Build history of the part. All positions in model axes, mm. Face numbers are marked on the shaded views. A direction names the side the tool comes from. Round coordinates to 2 decimals unless told otherwise and drop trailing zeros. Write each loop counter-clockwise with the first axis right and the second up, starting at its lowest first coordinate (ties: lowest second). Pieces come first, ordered by that corner, then holes.
Item 1: Band-saw the part on C-C, the plane x = -3. Write the cut outline in (y, z).
Item 2: Band-saw the part on A-A, the plane y = -2. Write the cut outline in (x, z).
Item 3: Wall check: probe 1 along Y at (x, z) = (0, 53.75); probe 2 along X at (y, z) = (0, 55.5); probe 3 along Z at (x, y) = (5.5, 1.25). Give the ranges that are in metal, low to high.
Item 4: 3-axis set-ups, long thin cutter, end or side, ignore diameter. For the marked faces 1 and 2: which of +Z, -Z, +X, -X, +Y, -Y reach the whole face in a straight line?
Item 5: Drop flat-ended pins along their axis: pin 1 Ø1 at (y, z) = (0.5, 33) entering from +X; pin 2 Ø1.5 at (y, z) = (5, 49) entering from -X; pin 3 Ø2 at (y, z) = (-2, 10.5) entering from -X. Give the stop position or say it passes through.
Item 6: Band-saw the part on B-B, the plane z = 13. Write the cut outline in (x, y), then the cut area to 3 significant figures.
Autodesk Inventor part; units mm, degrees
ref_plane "作業平面1" through (0, 6, 58.85) normal (0, 1, 0) x (-1, 0, 0)
ref_plane "YZ Plane" through (0, 0, 0) normal (1, 0, 0) x (0, 1, 0)
ref_plane "XZ Plane" through (0, 0, 0) normal (0, 1, 0) x (-1, 0, 0)
sketch "スケッチ1" plane through (0, 0, 0) normal (0, 0, 1) x (1, 0, 0)
  point P0 (0, 0)
sketch "スケッチ2" plane through (0, 0, 0) normal (0, 0, 1) x (1, 0, 0)
  circle A0 centre (0, 0) radius 5
  dimension "d0" = 10
extrude "押し出し1" add sketch "スケッチ2" along normal blind 35
thread "ねじ1"
sketch "スケッチ3" plane through (0, 0, 35) normal (0, 0, 1) x (1, 0, 0)
  point P0 (0, 0)
sketch "スケッチ4" plane through (0, 0, 35) normal (0, 0, 1) x (1, 0, 0)
  circle A0 centre (0, 0) radius 6
  dimension "d5" = 12
extrude "押し出し2" add sketch "スケッチ4" along normal blind 23.85
sketch "スケッチ5" plane through (0, 0, 58.85) normal (0, 0, 1) x (1, 0, 0)
  line L0 (0, 0) -> (0, 6)
  circle A0 centre (0, 0) radius 6
ref_plane "作業平面1" through (0, 6, 58.85) normal (0, 1, 0) x (-1, 0, 0)
sketch "スケッチ6" plane through (0, 6, 58.85) normal (0, 1, 0) x (-1, 0, 0)
  line L0 (6, 0) -> (-6, 0)
  line L1 (-2, 0) -> (2, 0)
  line L2 (2, 0) -> (2, -13)
  line L3 (-2, -13) -> (-2, 0)
  arc A0 (-2, -13) -> (2, -13) centre (0, -13) ccw
  point P0 (0, -58.85)
  point P1 (0, 0)
  dimension "d8" = 2
  dimension "d9" = 2
  dimension "d12" = 4
extrude "押し出し3" cut sketch "スケッチ6" against normal blind 2.157
sketch "スケッチ7" plane through (0, 0, 58.85) normal (0, 0, 1) x (1, 0, 0)
  point P0 (0, 0)
  point P1 (0, 0)
hole "穴1" at (0, 0, 58.85) direction (0, 0, -1) diameter 3 depth 8 tip angle 118
thread "ねじ2"
properties part number "回転アーム付き計測輪シャフト"
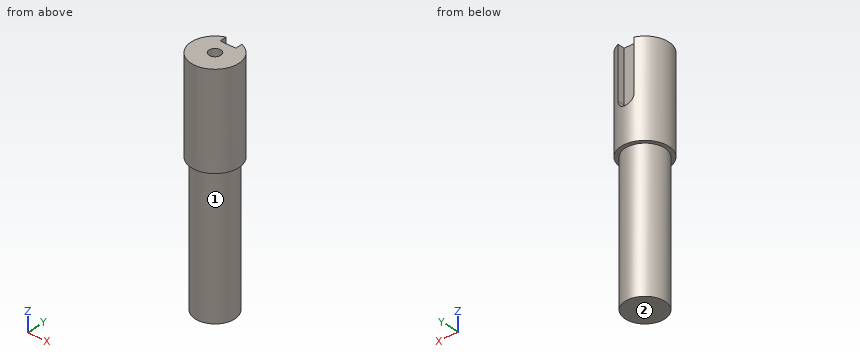
Results:
1. outline: (-5.2, 35) - (-4, 35) - (-4, 0) - (4, 0) - (4, 35) - (5.2, 35) - (5.2, 58.85) - (-5.2, 58.85) - close
2. outline: (-5.66, 35) - (-4.58, 35) - (-4.58, 0) - (4.58, 0) - (4.58, 35) - (5.66, 35) - (5.66, 58.85) - (-5.66, 58.85) - close
3. probe 1: y = -6 to -1.5, 1.5 to 3.84
3. probe 2: x = -6 to -1.5, 1.5 to 6
3. probe 3: z = 35 to 58.85
4. face 1: -Z
4. face 2: -Z, +X, -X, +Y, -Y
5. pin 1: stops at x = 5
5. pin 2: stops at x = -4.24
5. pin 3: stops at x = -4.9
6. outline: circle Ø10 at (0, 0)
6. area: 78.5 mm2
